The listing builds one solid part. Answer for the finished solid, in the listing's coordinates (mm). A direction names the side the tool comes from. Coordinates: 2 decimals unless noted, no trailing zeros. Loops run counter-clockwise (first coordinate to the right, second up) from the corner with the lowest first, then second, coordinate; pieces in that order, holes last. Notation, with made-up numbers: (-33, 61.25) - (15, 61.25) arc R22 ccw to (15, 96.25) - close; hole circle Ø9 at (-14.75, -25.5). An arc over 180 degrees is marked (long way). One line per question, with ' | ' between items.
from build123d import *

# Parameters (mm, degrees)
F0_R     = 40
F1_DEPTH = 3
F2_R     = 5
F3_DEPTH = 25
F4_R     = 25
F5_DEPTH = 3


with BuildPart() as f1:
    # F0 (on Top) → F1 (new body)
    with BuildSketch(Plane.XY):
        Circle(F0_R)
    extrude(amount=-F1_DEPTH)

    # F2 (on Top) → F3 (cut)
    with BuildSketch(Plane.XY):
        with Locations((0, 32.5)):
            Circle(F2_R)
        with Locations((-28.145826, -16.25)):
            Circle(F2_R)
        with Locations((28.145826, -16.25)):
            Circle(F2_R)
    extrude(amount=-F3_DEPTH, mode=Mode.SUBTRACT)

    # F4 (on face) → F5 (join)
    with BuildSketch(Plane(origin=(0, 0, -3), x_dir=(1, 0, 0), z_dir=(0, 0, -1))):
        Circle(F4_R)
    extrude(amount=F5_DEPTH)


solid = f1.part
Item 1: Find section B-B, the plane y = -16.25. Write down the section's boundary in (x, z).
Taken from the geometry:
outline: (-36.55, -3) - (-33.15, -3) - (-33.15, 0) - (-36.55, 0) - close; (-23.15, -3) - (-19, -3) - (-19, -6) - (19, -6) - (19, -3) - (23.15, -3) - (23.15, 0) - (-23.15, 0) - close; (33.15, -3) - (36.55, -3) - (36.55, 0) - (33.15, 0) - close
Item 2: The mould has two halves that part along Y. Classify faces 1 (the face through (-8.67, -39.05, -1.48)), 2 (the face through (-25.839, -20.686, -1.479)), 3 (the face through (-1, 1, 0)): pulls with the +Y half, pulls with the -Y half, needs draft (parallel to the pull), parting line crosses it, or undercut.
Taken from the geometry:
face 1: parting line crosses it | face 2: undercut | face 3: needs draft
Item 3: Each of these flat-tipped pins is pushed along its axis until it touches: pin 1 Ø1.5 at (y, z) = (4.5, -4) entering from -X; pin 2 Ø5 at (x, y) = (-23.5, 22) entering from -Z; pin 3 Ø3 at (x, z) = (4, -2.5) entering from +Y. Where does it stop, or does it pass through?
Taken from the geometry:
pin 1: stops at x = -24.72 | pin 2: stops at z = -3 | pin 3: stops at y = 39.92
Item 4: Find section D-D, the plane x = -8. Write down the section's boundary in (y, z), plus the area to 3 significant figures.
Taken from the geometry:
outline: (-39.19, -3) - (-23.69, -3) - (-23.69, -6) - (23.69, -6) - (23.69, -3) - (39.19, -3) - (39.19, 0) - (-39.19, 0) - close | area: 377 mm2
Item 5: Find section C-C, the plane y = 0. Write down the section's boundary in (x, z).
Taken from the geometry:
outline: (-40, -3) - (-25, -3) - (-25, -6) - (25, -6) - (25, -3) - (40, -3) - (40, 0) - (-40, 0) - close
Item 6: Find the intervals of material crossed by line 1 (Y direction, x = 0, z = -0.9); line 2 (Z direction, x = -24, y = -30.5); line 3 (Y direction, x = -3.5, z = -2.85), in increasing order. Write a range as [from, to].
Taken from the geometry:
line 1: y = [-40, 27.5], [37.5, 40] | line 2: z = [-3, 0] | line 3: y = [-39.85, 28.93], [36.07, 39.85]
Item 7: Find section A-A, the plane x = 0. Write down the section's boundary in (y, z), plus the area to 3 significant figures.
Taken from the geometry:
outline: (-40, -3) - (-25, -3) - (-25, -6) - (25, -6) - (25, -3) - (27.5, -3) - (27.5, 0) - (-40, 0) - close; (37.5, -3) - (40, -3) - (40, 0) - (37.5, 0) - close | area: 360 mm2
Item 8: Which of the six approach directions +Z, -Z, +X, -X, +Y, -Y give full straight-line access (tool end or side, diameter ignored) to faces 4 (the face through (32.765, -18.165, -1.479)), 5 (the face through (17.22, 18.34, -3))?
Taken from the geometry:
face 4: +Z, -Z | face 5: -Z
